```python
from build123d import *

# Parameters (mm, degrees)
CROQUIS1_R              = 10
SALIENTE_EXTRUIR1_DEPTH = 2
CROQUIS4_R              = 8
SALIENTE_EXTRUIR2_DEPTH = 3
CROQUIS5_R              = 10
SALIENTE_EXTRUIR3_DEPTH = 2
CHAFL_N1_SIZE           = 1
CHAFL_N2_SIZE           = 1
CROQUIS7_R              = 4
SALIENTE_EXTRUIR4_DEPTH = 4
CORTAR_EXTRUIR1_DEPTH   = 16.779733838
CROQUIS8_R              = 1
CORTAR_EXTRUIR2_DEPTH   = 18.916472867
CROQUIS9_R              = 2.5
CORTAR_EXTRUIR3_DEPTH   = 5


with BuildPart() as part:
    # Croquis1 → Saliente-Extruir1 (new body)
    with BuildSketch(Plane(origin=(0, 0, 0), x_dir=(1, 0, 0), z_dir=(0, 1, 0))):
        with Locations(Location((0, 0, 0), (0, 0, 270))):
            Circle(CROQUIS1_R)
    extrude(amount=SALIENTE_EXTRUIR1_DEPTH)

    # Croquis4 → Saliente-Extruir2 (add)
    with BuildSketch(Plane(origin=(0, 2, 0), x_dir=(1, 0, 0), z_dir=(0, 1, 0))):
        with Locations(Location((0, 0, 0), (0, 0, 270))):
            Circle(CROQUIS4_R)
    extrude(amount=SALIENTE_EXTRUIR2_DEPTH)

    # Croquis5 → Saliente-Extruir3 (add)
    with BuildSketch(Plane(origin=(0, 5, 0), x_dir=(1, 0, 0), z_dir=(0, 1, 0))):
        with Locations(Location((0, 0, 0), (0, 0, 270))):
            Circle(CROQUIS5_R)
    extrude(amount=SALIENTE_EXTRUIR3_DEPTH)

    # Chaflán1
    chafl_n1_edges = [part.edges().sort_by_distance(p)[0] for p in [
        (0, 7, -10),
    ]]
    chamfer(chafl_n1_edges, length=CHAFL_N1_SIZE)

    # Chaflán2
    chafl_n2_edges = [part.edges().sort_by_distance(p)[0] for p in [
        (0, 0, -10),
    ]]
    chamfer(chafl_n2_edges, length=CHAFL_N2_SIZE)

    # Croquis7 → Saliente-Extruir4 (add)
    with BuildSketch(Plane(origin=(0, 7, 0), x_dir=(1, 0, 0), z_dir=(0, 1, 0))):
        with Locations(Location((0, 0, 0), (0, 0, 270))):
            Circle(CROQUIS7_R)
    extrude(amount=SALIENTE_EXTRUIR4_DEPTH)

    # Croquis6 → Cortar-Extruir1 (cut, through all)
    with BuildSketch(Plane(origin=(0, 7, 0), x_dir=(1, 0, 0), z_dir=(0, 1, 0))):
        with BuildLine():
            Line((-1.653594569, -1.875), (1.653594569, -1.875))
            ThreePointArc((1.653594569, -1.875), (2.5, 0), (1.653594569, 1.875))
            Line((1.653594569, 1.875), (-1.653594569, 1.875))
            ThreePointArc((-1.653594569, 1.875), (-2.5, 0), (-1.653594569, -1.875))
        make_face()
    extrude(amount=CORTAR_EXTRUIR1_DEPTH, mode=Mode.SUBTRACT)

    # Croquis8 → Cortar-Extruir2 (cut, through all)
    with BuildSketch(Plane.XZ):
        with Locations(Location((0, 0, 0), (0, 0, 270))):
            Circle(CROQUIS8_R)
    extrude(amount=-CORTAR_EXTRUIR2_DEPTH, mode=Mode.SUBTRACT)

    # Croquis9 → Cortar-Extruir3 (cut)
    with BuildSketch(Plane.XZ):
        with Locations(Location((0, 0, 0), (0, 0, 270))):
            Circle(CROQUIS9_R)
    extrude(amount=-CORTAR_EXTRUIR3_DEPTH, mode=Mode.SUBTRACT)


solid = part.part
```
The model under review builds one solid part; all positions refer to its coordinate system, in mm. A direction names the side the tool comes from. Round coordinates to 2 decimals unless told otherwise and drop trailing zeros. Loops run counter-clockwise (first coordinate to the right, second up) from the corner with the lowest first, then second, coordinate; pieces in that order, holes last.
1) Wall thickness on line 1 along Y through (x, z) = (8.5, 1); line 2 along X through (y, z) = (5.7, 0); line 3 along Y through (x, z) = (-3, 2.75): over which ranges is each line inside the solid? List them lowest first.
Values follow:
line 1: y = 0 to 2, 5 to 7
line 2: x = -10 to -1, 1 to 10
line 3: y = 0 to 7
2) Tool access review of faces 5 (the face through (-1, 7, -1)), 6 (the face through (-2.44, 2.46, 0.54)), 7 (the face through (8.2, 5, 0)): name each direction out of +Z, -Z, +X, -X, +Y, -Y from which nothing blocks a thin tool from reaching the whole face with its end or side.
Values follow:
face 5: +Y
face 6: -Y
face 7: none
3) Consider section C-C on y = 8.5. State the section outline as (x, z) points (3 decimals).
Values follow:
outline: circle Ø8 at (0, 0); hole (-1.654, -1.875) - (1.654, -1.875) arc R2.5 ccw to (1.654, 1.875) - (-1.654, 1.875) arc R2.5 ccw to start
4) Consider section D-D on y = 5.25. State the section outline as (x, z) points, then the cut area to 3 significant figures.
Values follow:
outline: circle Ø20 at (0, 0); hole circle Ø2 at (0, 0)
area: 311 mm2
5) The part is to be moulded in two halves that separate along Z. For faces 1 (the face through (2.5, 9, 0)), 2 (the face through (0, 9, -1.875)), 3 (the face through (-7.81, 3.48, -1.73)), 4 (the face through (8.2, 2, 0)), say which applies: pulls with the +Z half, pulls with the -Z half, needs draft (parallel to the pull), parting line crosses it, or undercut.
Values follow:
face 1: undercut
face 2: undercut
face 3: parting line crosses it
face 4: needs draft
6) Clearance check with flat-ended pins moving along their axes: P1, Ø1.7, axis at x = -0.5, y = 8, coming from the -Z side; P2, Ø3, axis at x = -7, z = 6, coming from the +Y side; P3, Ø1, axis at x = -2, y = 1, coming from the -Z side. State where each tip first meets the part, or that it passes through.
Values follow:
P1: stops at z = -4
P2: stops at y = 7
P3: stops at z = -9.89
